Job drawing, mm, ordinate dimensions from the low corner. One solid piece. A direction names the side the tool comes from. Give positions to 0.01 mm unless a question says otherwise; leave off trailing zeros. Order: outer loops, then holes, each group sorted by start corner. A loop starts at its lowest first (then second) coordinate and runs counter-clockwise, first axis right, second up. Notation, with made-up numbers: M -3,21 L 42,21 A12 ccw 42,37 Z; hole C -39,79 d11. An arc over 180 degrees is marked long. One line per item, written item: value. Start each with the question number.
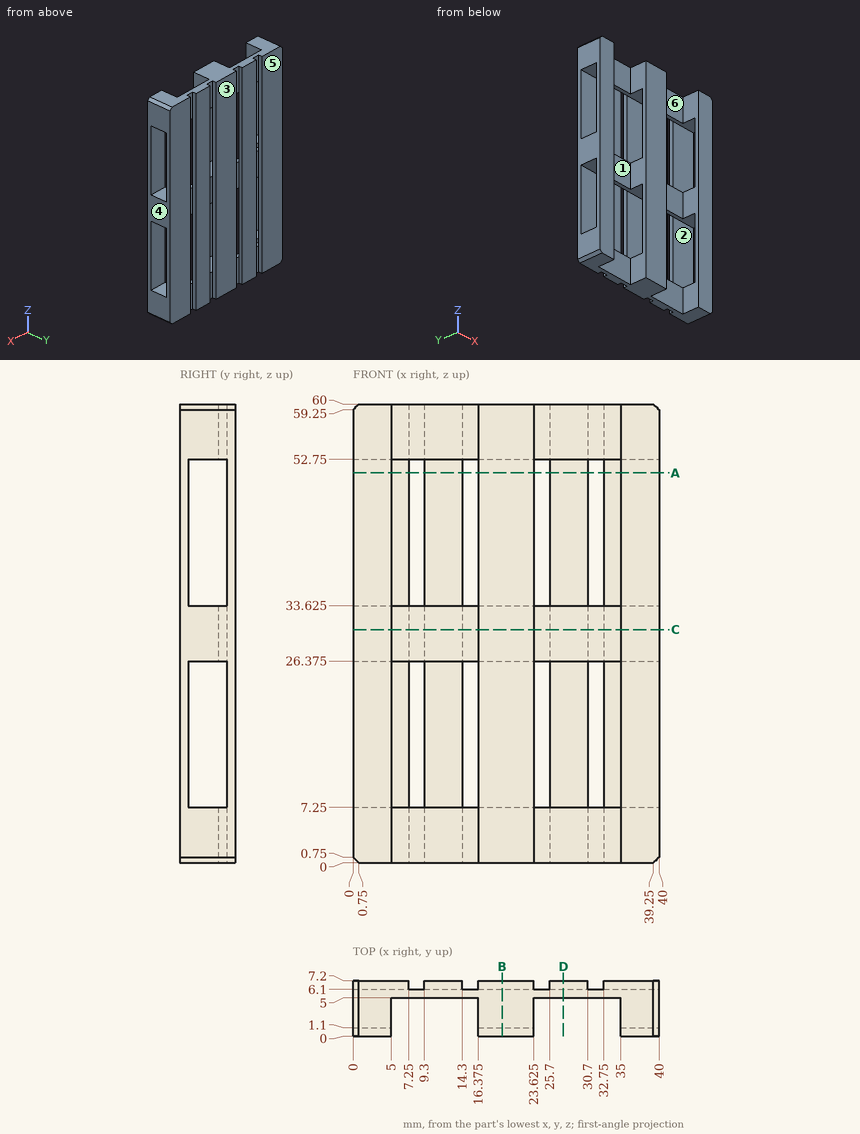
1) Drop flat-ended pins along their axis: P1, Ø0.6, axis at x = 32, z = 4, coming from the +Y side; P2, Ø5, axis at x = 32, z = 26, coming from the -Y side. Give the stop position or say it passes through.
2) Tool access for the marked faces 1, 2 and 3: list every direction of +Z, -Z, +X, -X, +Y, -Y with a clear straight run to the whole face (end or side of a thin tool).
3) Drill centre lines: line 1 (Z direction, x = 4, y = 1.75) (3 decimals); line 2 (X direction, y = 0.5, z = 4) (3 decimals); line 3 (X direction, y = 6.75, z = 54.5) (3 decimals). Where is each one in solid material? Low to high.
4) Slice it at B-B (x = 19.5). List the corners of the cut face in (y, z) (3 decimals), plus the area to 3 significant figures.
5) Slice it at C-C (z = 30.5). List the corners of the cut face in (x, y) (3 decimals).
6) Slice it at A-A (z = 51). State how many separate pieces and enclosed holes the cut face has, plus the area to 3 significant figures.
7) Slice it at D-D (x = 27.5). List the corners of the cut face in (y, z) (3 decimals).
8) Pull direction X, two halves, no side cores. Call the marked faces 4, 5 and 6: pulls with the +X half, pulls with the -X half, needs draft (parallel to the pull), parting line crosses it, or undercut.
Results list:
1. P1: stops at y = 6.1
1. P2: stops at y = 5
2. face 1: +Z, -Z, -Y
2. face 2: +X, -X
2. face 3: +Z, -Z, +X, -X, +Y
3. line 1: z = 0 to 7.25, 26.375 to 33.625, 52.75 to 60
3. line 2: x = 0 to 5, 16.375 to 23.625, 35 to 40
3. line 3: x = 0 to 7.25, 9.3 to 14.3, 16.375 to 23.625, 25.7 to 30.7, 32.75 to 40
4. outline: M 0,0 L 7.2,0 L 7.2,60 L 0,60 Z; hole M 1.1,7.25 L 6.1,7.25 L 6.1,26.375 L 1.1,26.375 Z; hole M 1.1,33.625 L 6.1,33.625 L 6.1,52.75 L 1.1,52.75 Z
4. area: 241 mm²
5. outline: M 0,0 L 5,0 L 5,5 L 16.375,5 L 16.375,0 L 23.625,0 L 23.625,5 L 35,5 L 35,0 L 40,0 L 40,7.2 L 32.75,7.2 L 32.75,6.1 L 30.7,6.1 L 30.7,7.2 L 25.7,7.2 L 25.7,6.1 L 23.625,6.1 L 23.625,7.2 L 16.375,7.2 L 16.375,6.1 L 14.3,6.1 L 14.3,7.2 L 9.3,7.2 L 9.3,6.1 L 7.25,6.1 L 7.25,7.2 L 0,7.2 Z
6. separate pieces: 8
6. enclosed holes: 0
6. area: 53.9 mm²
7. outline: M 5,0 L 7.2,0 L 7.2,60 L 5,60 L 5,52.75 L 6.1,52.75 L 6.1,33.625 L 5,33.625 L 5,26.375 L 6.1,26.375 L 6.1,7.25 L 5,7.25 Z
8. face 4: pulls with the +X half
8. face 5: needs draft
8. face 6: undercut
